from build123d import *

# Parameters (mm, degrees)
SKETCH1_R           = 4.729578235
SKETCH1_R_2         = 1.475
SKETCH1_R_3         = 2
SKETCH1_R_4         = 2.75
BOSS_EXTRUDE1_DEPTH = 4


with BuildPart() as part:
    # Sketch1 → Boss-Extrude1 (new body)
    # profile 1 of 3: a face of its own
    with BuildSketch(Plane(origin=(0, 0, 0), x_dir=(1, 0, 0), z_dir=(0, 1, 0))):
        with Locations((0, 45)):
            Circle(SKETCH1_R)
        with Locations(Location((0, 45, 0), (0, 0, 270))):
            Circle(SKETCH1_R_2, mode=Mode.SUBTRACT)
    # profile 2 of 3: a face of its own
    with BuildSketch(Plane(origin=(0, 0, 0), x_dir=(1, 0, 0), z_dir=(0, 1, 0))):
        with BuildLine():
            Line((11.849111677, 4.273338853), (4.729578235, 45))
            ThreePointArc((4.729578235, 45), (0, 40.270421765), (-4.729578235, 45))
            Line((-4.729578235, 45), (-11.849111677, 4.273338853))
            ThreePointArc((-11.849111677, 4.273338853), (0, 12.596145144), (11.849111677, 4.273338853))
        make_face()
    # profile 3 of 3: a face of its own
    with BuildSketch(Plane(origin=(0, 0, 0), x_dir=(1, 0, 0), z_dir=(0, 1, 0))):
        with BuildLine():
            Line((12.596145144, 0), (11.849111677, 4.273338853))
            ThreePointArc((11.849111677, 4.273338853), (0, 12.596145144), (-11.849111677, 4.273338853))
            Line((-11.849111677, 4.273338853), (-12.596145144, 0))
            ThreePointArc((-12.596145144, 0), (0, -12.596145144), (12.596145144, 0))
        make_face()
        with Locations(Location((-6.35, 0, 0), (0, 0, 270))):
            Circle(SKETCH1_R_3, mode=Mode.SUBTRACT)
        with Locations(Location((0, -6.35, 0), (0, 0, 270))):
            Circle(SKETCH1_R_3, mode=Mode.SUBTRACT)
        with Locations(Location((0, 0, 0), (0, 0, 270))):
            Circle(SKETCH1_R_4, mode=Mode.SUBTRACT)
        with Locations(Location((6.35, 0, 0), (0, 0, 270))):
            Circle(SKETCH1_R_3, mode=Mode.SUBTRACT)
        with Locations(Location((0, 6.35, 0), (0, 0, 270))):
            Circle(SKETCH1_R_3, mode=Mode.SUBTRACT)
    extrude(amount=BOSS_EXTRUDE1_DEPTH)


solid = part.part
The listing builds one solid part. Answer for the finished solid, in the listing's coordinates (mm). Round coordinates to 2 decimals unless told otherwise and drop trailing zeros. Order: outer loops, then holes, each group sorted by start corner. A loop starts at its lowest first (then second) coordinate and runs counter-clockwise, first axis right, second up. Notation, with made-up numbers: (-29, -21.75) -> (16, -21.75) arc R25 cw to (16, -2.75) -> close; hole circle Ø6 at (65, -4.5). An arc over 180 degrees is marked (long way). Write each question's results on one line, items separated by ' | '. Start each with the question number.
Q1. Find section D-D (z = -16.5). Determine the outline of the cut face in (x, y), then the cut area to 3 significant figures.
Q2. Straight lines are drawn through the part: probe 1 along X at (y, z) = (1.65, 0); probe 2 along X at (y, z) = (0.65, -1); probe 3 along Z at (x, y) = (0.25, 0.35). For each, find the intervals that lie inside material, in ascending order. Write a range as from..to.
Q3. The mould has two halves that part along Z. Classify faces 1 (the cylindrical face through (-0.277, 1.972, 12.593)), 2 (the cylindrical face through (-1.217, 1.972, -7.937)), 3 (the cylindrical face through (0.1, 1.97, -49.73)): pulls with the +Z half, pulls with the -Z half, needs draft (parallel to the pull), parting line crosses it, or undercut.
Q4. Find section C-C (z = 6.35). Determine the outline of the cut face in (x, y), then the cut area to 3 significant figures.
Q5. Each of these flat-tipped pins is pushed along its axis until it touches: pin 1 (1 mm diameter, centred on y = 3.5, z = -8.5, fed in from -X); pin 2 (5 mm diameter, centred on x = 2, z = -2.5, fed in from -Y); pin 3 (1 mm diameter, centred on x = 5.5, y = 3.5, fed in from +Z); pin 4 (1 mm diameter, centred on x = -8.5, y = 0.5, fed in from +Z). Where does it stop, or does it pass through?
Q6. Find section B-B (x = -7). Determine the outline of the cut face in (y, z).
Q7. Find section A-A (y = 3.2). Determine the outline of the cut face in (x, z) (3 decimals).
Worked answers:
1) outline: (-9.71, 0) -> (9.71, 0) -> (9.71, 4) -> (-9.71, 4) -> close | area: 77.7 mm2
2) probe 1: x = -12.6..-8.35, -4.35..-2.75, 2.75..4.35, 8.35..12.6 | probe 2: x = -12.42..-8.08, -4.62..-2.56, 2.56..4.62, 8.08..12.42 | probe 3: z = -49.72..-46.45, -43.55..-8.33, -4.37..-2.74, 2.74..4.37, 8.33..12.59
3) face 1: pulls with the +Z half | face 2: undercut | face 3: pulls with the -Z half
4) outline: (-10.88, 0) -> (-2, 0) -> (-2, 4) -> (-10.88, 4) -> close; (2, 0) -> (10.88, 0) -> (10.88, 4) -> (2, 4) -> close | area: 71.0 mm2
5) pin 1: stops at x = -11.2 | pin 2: stops at y = 0 | pin 3: stops at z = 11.56 | pin 4: stops at z = 9.73
6) outline: (0, -32.01) -> (4, -32.01) -> (4, -1.89) -> (0, -1.89) -> close; (0, 1.89) -> (4, 1.89) -> (4, 10.47) -> (0, 10.47) -> close
7) outline: (-12.596, 0) -> (-4.73, -45) arc R4.73 ccw to (4.73, -45) -> (12.596, 0) arc R12.596 ccw to start; hole circle Ø4 at (-6.35, 0); hole circle Ø5.5 at (0, 0); hole circle Ø4 at (0, -6.35); hole circle Ø4 at (0, 6.35); hole circle Ø2.95 at (0, -45); hole circle Ø4 at (6.35, 0)
